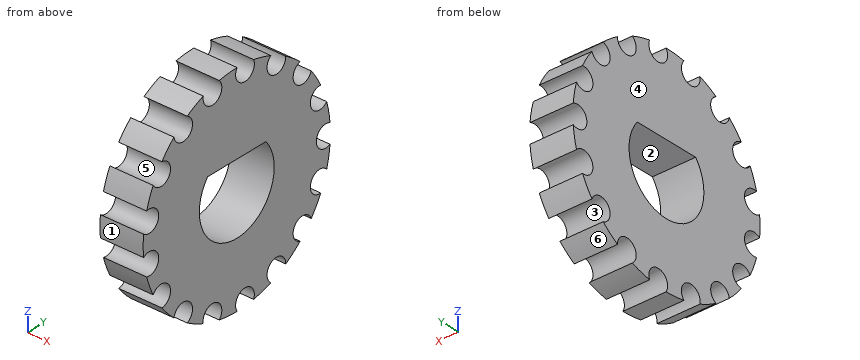
from build123d import *

# Parameters (mm, degrees)
SKETCH_1_R          = 10
EXTRUDE_2_DEPTH     = 4
SKETCH_2_R          = 1
CUT_EXTRUDE_1_DEPTH = 4
CUT_EXTRUDE_2_DEPTH = 4


with BuildPart() as part:
    # Эскиз1 → Бобышка-Вытянуть2 (new body)
    with BuildSketch(Plane(origin=(0, 0, 0), x_dir=(0, 0, -1), z_dir=(1, 0, 0))):
        Circle(SKETCH_1_R)
    extrude(amount=EXTRUDE_2_DEPTH)

    # Эскиз2 → Вырез-Вытянуть1 (cut)
    with BuildSketch(Plane.ZY):
        with Locations((0, 9.5)):
            Circle(SKETCH_2_R)
        with Locations((3.431795829, 8.858486179)):
            Circle(SKETCH_2_R)
        with Locations((6.400108615, 7.020584714)):
            Circle(SKETCH_2_R)
        with Locations((8.504051268, 4.23451438)):
            Circle(SKETCH_2_R)
        with Locations((9.459474675, 0.876549415)):
            Circle(SKETCH_2_R)
        with Locations((9.13734361, -2.599798406)):
            Circle(SKETCH_2_R)
        with Locations((7.581163659, -5.725029046)):
            Circle(SKETCH_2_R)
        with Locations((5.001105547, -8.077062789)):
            Circle(SKETCH_2_R)
        with Locations((1.745620419, -9.338244447)):
            Circle(SKETCH_2_R)
        with Locations((-1.745620419, -9.338244447)):
            Circle(SKETCH_2_R)
        with Locations((-5.001105547, -8.077062789)):
            Circle(SKETCH_2_R)
        with Locations((-7.581163659, -5.725029046)):
            Circle(SKETCH_2_R)
        with Locations((-9.13734361, -2.599798406)):
            Circle(SKETCH_2_R)
        with Locations((-9.459474675, 0.876549415)):
            Circle(SKETCH_2_R)
        with Locations((-8.504051268, 4.23451438)):
            Circle(SKETCH_2_R)
        with Locations((-6.400108615, 7.020584714)):
            Circle(SKETCH_2_R)
        with Locations((-3.431795829, 8.858486179)):
            Circle(SKETCH_2_R)
    extrude(amount=-CUT_EXTRUDE_1_DEPTH, mode=Mode.SUBTRACT)

    # Эскиз3 → Вырез-Вытянуть2 (cut)
    with BuildSketch(Plane(origin=(4, 0, 0), x_dir=(0, 0, -1), z_dir=(1, 0, 0))):
        with BuildLine():
            Line((-2.5, 3.122498999), (-2.5, -3.122498999))
            ThreePointArc((-2.5, -3.122498999), (4, 0), (-2.5, 3.122498999))
        make_face()
    extrude(amount=-CUT_EXTRUDE_2_DEPTH, mode=Mode.SUBTRACT)


solid = part.part
Geometry: final body of the model. Coordinates: model frame, mm. Face numbers are marked on the shaded views. A direction names the side the tool comes from. Coordinates: 2 decimals unless noted, no trailing zeros. Order: outer loops, then holes, each group sorted by start corner. A loop starts at its lowest first (then second) coordinate and runs counter-clockwise, first axis right, second up.
(1) Section query B-B (z = 0). Return the cut outline in (x, y), plus the area to 3 significant figures.
(2) Section query C-C (y = 7.25). Return the cut outline in (x, z), plus the area to 3 significant figures.
(3) Access query for the marked faces 1 and 2. Directions: +Z, -Z, +X, -X, +Y, -Y. A direction counts if a zero-diameter tool reaches every point of the face in a straight line with its end or side. Return the directions, or none.
(4) First-contact query: pin 1 (1.2 mm diameter, centred on y = -5.73, z = -7.58, fed in from +X); pin 2 (7 mm diameter, centred on y = 0, z = 0, fed in from -X); pin 3 (1 mm diameter, centred on x = 3, z = -6, fed in from -Y); pin 4 (2 mm diameter, centred on x = 1, y = 3, fed in from -Z). Flat tips, straight axial feed; report the tip coordinate or a pass-through.
(5) Section query A-A (z = -3). Return the cut outline in (x, y).
(6) Draft query along Y for the marked faces 3, 4, 5 and 6. Return one class per face: pulls with the +Y half, pulls with the -Y half, needs draft (parallel to the pull), parting line crosses it, or undercut.
(7) Material intervals for probe 1 along Y at (x, z) = (1.3, 8.25); probe 2 along Z at (x, y) = (1.1, -8.5); probe 3 along Z at (x, y) = (2, 7), sorted ascending.
Solution:
1. outline: (0, -10) - (4, -10) - (4, -4) - (0, -4) - close; (0, 4) - (4, 4) - (4, 8.5) - (0, 8.5) - close
1. area: 42.0 mm2
2. outline: (0, -5.43) - (4, -5.43) - (4, 5.43) - (0, 5.43) - close
2. area: 43.4 mm2
3. face 1: +X, -X, -Y
3. face 2: +X, -X
4. pin 1: passes through
4. pin 2: stops at x = 0
4. pin 3: stops at y = -8
4. pin 4: stops at z = -9.8
5. outline: (0, -9.54) - (4, -9.54) - (4, -2.65) - (0, -2.65) - close; (0, 2.65) - (4, 2.65) - (4, 7.96) - (0, 7.96) - close
6. face 3: undercut
6. face 4: needs draft
6. face 5: undercut
6. face 6: pulls with the +Y half
7. probe 1: y = -4.98 to -3.06, -2.14 to 3.27, 5.2 to 5.65
7. probe 2: z = -4.09 to -2.29, -1.2 to 1.2, 2.29 to 4.09
7. probe 3: z = -5.4 to 5.4
